```python
from build123d import *

# Parameters (mm, degrees)
SKETCH1_W           = 40
SKETCH1_H           = 20
BOSS_EXTRUDE1_DEPTH = 1.44
SKETCH2_R           = 2.5
BOSS_EXTRUDE2_DEPTH = 8.7
FILLET1_R           = 2
SKETCH3_R           = 1
CUT_EXTRUDE1_DEPTH  = 24.993540797


with BuildPart() as part:
    # Sketch1 → Boss-Extrude1 (new body)
    with BuildSketch(Plane(origin=(0, 0, 0), x_dir=(1, 0, 0), z_dir=(0, 1, 0))):
        Rectangle(SKETCH1_W, SKETCH1_H)
    extrude(amount=BOSS_EXTRUDE1_DEPTH)

    # Sketch2 → Boss-Extrude2 (add)
    with BuildSketch(Plane(origin=(0, 1.44, 0), x_dir=(1, 0, 0), z_dir=(0, 1, 0))):
        with Locations(Location((14.35, 4.9, 0), (0, 0, 90))):
            Circle(SKETCH2_R)
        with Locations(Location((-0.89, 4.9, 0), (0, 0, 90))):
            Circle(SKETCH2_R)
        with Locations(Location((-16.13, 4.9, 0), (0, 0, 90))):
            Circle(SKETCH2_R)
    extrude(amount=BOSS_EXTRUDE2_DEPTH)

    # Fillet1
    fillet1_edges = [part.edges().sort_by_distance(p)[0] for p in [
        (14.35, 10.14, -2.4),
        (-0.89, 10.14, -2.4),
        (-16.13, 10.14, -2.4),
    ]]
    fillet(fillet1_edges, radius=FILLET1_R)

    # Sketch3 → Cut-Extrude1 (cut, through all)
    with BuildSketch(Plane(origin=(0, 1.44, 0), x_dir=(1, 0, 0), z_dir=(0, 1, 0))):
        with Locations(Location((17.95, 7.95, 0), (0, 0, 270))):
            Circle(SKETCH3_R)
        with Locations(Location((17.95, -7.95, 0), (0, 0, 270))):
            Circle(SKETCH3_R)
    extrude(amount=-CUT_EXTRUDE1_DEPTH, mode=Mode.SUBTRACT)


solid = part.part
```
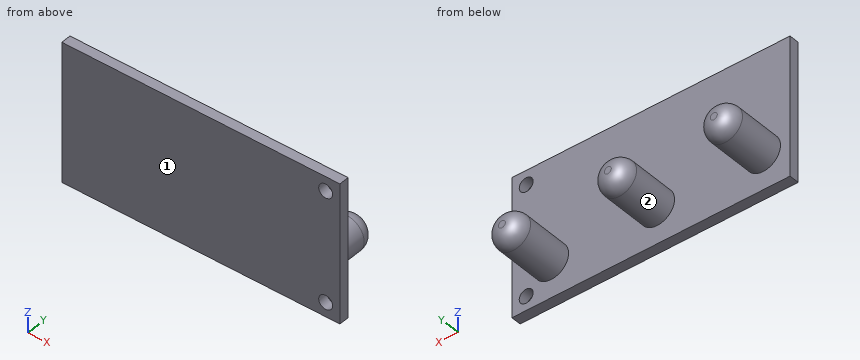
The listing builds one solid part. Answer for the finished solid, in the listing's coordinates (mm). Face numbers are marked on the shaded views. Give positions to 0.01 mm unless a question says otherwise; leave off trailing zeros. Order: outer loops, then holes, each group sorted by start corner. A loop starts at its lowest first (then second) coordinate and runs counter-clockwise, first axis right, second up. Notation, with made-up numbers: (48.5, -34.5) -> (58.5, -34.5) arc R34 ccw to (58.5, 2.5) -> close; hole circle Ø11 at (50, 46.5). An arc over 180 degrees is marked (long way). Answer as a JSON object with one key per item and string values. Group by question number.
Item 1: The part is cut by section D-D on z = 4. Write down the section's boundary in (x, y).
Item 2: The part is cut by section A-A on x = 17.95. Write down the section's boundary in (y, z), and give its area (3 significant figures).
Item 3: Consider L1, parallel to X at y = 8, z = -4.75; L2, parallel to X at y = 1.05, z = -7.95; L3, parallel to Y at x = 0, z = 5.75. Determine where each line is inside the solid, lowest interval first. Write a range as from..to.
Item 4: Determine the mould class of the marked faces 1 and 2 for opening direction X: pulls with the +X half, pulls with the -X half, needs draft (parallel to the pull), parting line crosses it, or undercut.
Item 5: The part is cut by section C-C on x = -10.5. Write down the section's boundary in (y, z), and give its area (3 significant figures).
Item 6: Flat-ended cylindrical pins translate along their axes: pin 1 (6 mm diameter, centred on x = 0.5, z = 2, fed in from +Y); pin 2 (2 mm diameter, centred on y = 4.5, z = -4, fed in from -X); pin 3 (2 mm diameter, centred on y = 4.5, z = -4, fed in from +X). Find the tip coordinate at first contact, or state that the pin passes through.
Item 7: The part is cut by section B-B on y = 6.25. Write down the section's boundary in (x, z), and give its area (3 significant figures).
Result set:
{
 "1": {"outline": "(-20, 0) -> (20, 0) -> (20, 1.44) -> (-20, 1.44) -> close"},
 "2": {"outline": "(0, -10) -> (1.44, -10) -> (1.44, -8.95) -> (0, -8.95) -> close; (0, -6.95) -> (1.44, -6.95) -> (1.44, 6.95) -> (0, 6.95) -> close; (0, 8.95) -> (1.44, 8.95) -> (1.44, 10) -> (0, 10) -> close", "area": "23.0 mm²"},
 "3": {"L1": "-18.63..-13.63, -3.39..1.61, 11.85..16.85", "L2": "-20..16.95, 18.95..20", "L3": "0..1.44"},
 "4": {"face 1": "needs draft", "face 2": "undercut"},
 "5": {"outline": "(0, -10) -> (1.44, -10) -> (1.44, 10) -> (0, 10) -> close", "area": "28.8 mm²"},
 "6": {"pin 1": "y = 1.44", "pin 2": "x = -18.63", "pin 3": "x = 16.85"},
 "7": {"outline": "circle Ø5 at (-16.13, -4.9); circle Ø5 at (-0.89, -4.9); circle Ø5 at (14.35, -4.9)", "area": "58.9 mm²"}
}
